For this review, use the dimensioned drawing (mm, ordinates from the lowest corner) and the shaded views. A direction names the side the tool comes from. Round coordinates to 2 decimals unless told otherwise and drop trailing zeros. Order: outer loops, then holes, each group sorted by start corner. A loop starts at its lowest first (then second) coordinate and runs counter-clockwise, first axis right, second up. Notation, with made-up numbers: (85.5, -36) - (130.5, -36) arc R28 ccw to (130.5, 3) - close; hole circle Ø6 at (34, 32.5). An arc over 180 degrees is marked (long way). Write item = value, one per line.
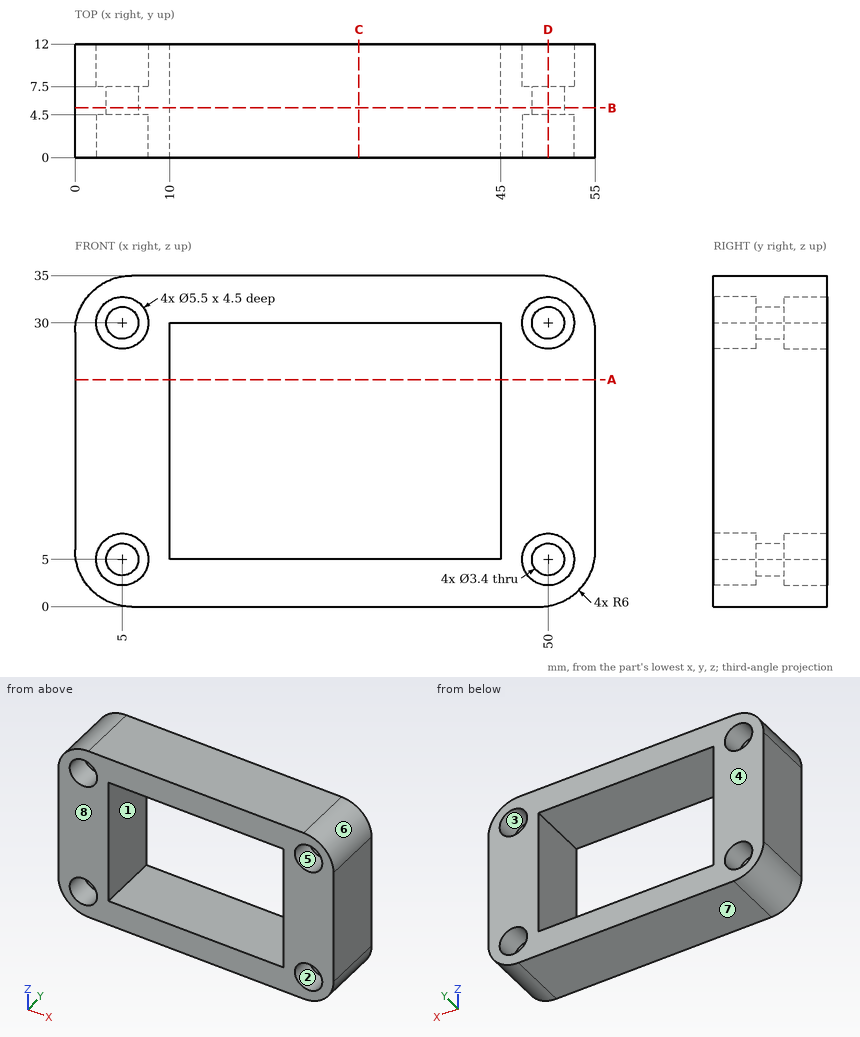
1) We need section A-A on z = 24. Write out the cut boundary in (x, y).
Findings:
outline = (0, 0) - (10, 0) - (10, 12) - (0, 12) - close; (45, 0) - (55, 0) - (55, 12) - (45, 12) - close
2) The part is to be moulded in two halves that separate along Z. For the marked faces 5, 6, 7 and 8, say which applies: released by +Z, released by -Z, zero draft, split by the parting line, or undercut.
Findings:
face_5 = undercut
face_6 = released by +Z
face_7 = released by -Z
face_8 = zero draft
3) We need section C-C on x = 30. Write out the cut boundary in (y, z), and give its area (3 significant figures).
Findings:
outline = (0, 0) - (12, 0) - (12, 5) - (0, 5) - close; (0, 30) - (12, 30) - (12, 35) - (0, 35) - close
area = 120 mm^2
4) For the marked faces 1, 2, 3 and 4, list the 3-axis set-ups (+Z, -Z, +X, -X, +Y, -Y) from which the entire face can be reached by the end or side of a thin tool; tool diameter is ignored.
Findings:
face_1 = +Y, -Y
face_2 = -Y
face_3 = +Y
face_4 = +Z, -Z, +X, -X, +Y
5) We need section D-D on x = 50. Write out the cut boundary in (y, z).
Findings:
outline = (0, 0.08) - (12, 0.08) - (12, 2.25) - (7.5, 2.25) - (7.5, 3.3) - (4.5, 3.3) - (4.5, 2.25) - (0, 2.25) - close; (0, 7.75) - (4.5, 7.75) - (4.5, 6.7) - (7.5, 6.7) - (7.5, 7.75) - (12, 7.75) - (12, 27.25) - (7.5, 27.25) - (7.5, 28.3) - (4.5, 28.3) - (4.5, 27.25) - (0, 27.25) - close; (0, 32.75) - (4.5, 32.75) - (4.5, 31.7) - (7.5, 31.7) - (7.5, 32.75) - (12, 32.75) - (12, 34.92) - (0, 34.92) - close
6) Clearance check with flat-ended pins moving along their axes: pin 1 Ø4.5 at (x, z) = (5, 30) entering from +Y; pin 2 Ø2 at (x, z) = (50, 5) entering from -Y; pin 3 Ø3 at (x, z) = (50, 6) entering from -Y; pin 4 Ø1.5 at (y, z) = (7.5, 4) entering from +X. State where each tip first meets the part, or that it passes through.
Findings:
pin_1 = 7.5
pin_2 = through
pin_3 = 4.5
pin_4 = 54.87
7) We need section B-B on y = 5.25. Write out the cut boundary in (x, z).
Findings:
outline = (0, 6) arc R6 ccw to (6, 0) - (49, 0) arc R6 ccw to (55, 6) - (55, 29) arc R6 ccw to (49, 35) - (6, 35) arc R6 ccw to (0, 29) - close; hole circle Ø3.4 at (5, 5); hole circle Ø3.4 at (5, 30); hole (10, 5) - (45, 5) - (45, 30) - (10, 30) - close; hole circle Ø3.4 at (50, 5); hole circle Ø3.4 at (50, 30)
8) To check wall thickness, follow L1, parallel to X at y = 10.75, z = 23; L2, parallel to Z at x = 5, y = 6.4; L3, parallel to Z at x = 12, y = 7.5. State the ranges of each line that lie inside material, in increasing order. Write a range as from..to.
Findings:
L1 = 0..10, 45..55
L2 = 0.08..3.3, 6.7..28.3, 31.7..34.92
L3 = 0..5, 30..35
